The model under review builds one solid part; all positions refer to its coordinate system, in mm. A direction names the side the tool comes from. Coordinates: 2 decimals unless noted, no trailing zeros. Order: outer loops, then holes, each group sorted by start corner. A loop starts at its lowest first (then second) coordinate and runs counter-clockwise, first axis right, second up. Notation, with made-up numbers: (-11.5, 63.5) - (0.5, 63.5) arc R29 cw to (0.5, 100.5) - close; hole circle Ø2 at (-33.75, 2). An arc over 180 degrees is marked (long way). Answer in a Markdown table with one row per item.
Autodesk Inventor part; units mm, degrees
ref_plane "YZ Plane" through (0, 0, 0) normal (1, 0, 0) x (0, 1, 0)
ref_plane "XZ Plane" through (0, 0, 0) normal (0, 1, 0) x (-1, 0, 0)
ref_plane "XY Plane" through (0, 0, 0) normal (0, 0, 1) x (1, 0, 0)
sketch "Sketch1" plane through (0, 0, 0) normal (0, 0, 1) x (1, 0, 0)
  line L0 (2.5, 1.4434) -> (2.5, -1.4434)
  line L1 (2.5, -1.4434) -> (0, -2.8868)
  line L2 (0, -2.8868) -> (-2.5, -1.4434)
  line L3 (-2.5, -1.4434) -> (-2.5, 1.4434)
  line L4 (-2.5, 1.4434) -> (0, 2.8868)
  line L5 (0, 2.8868) -> (2.5, 1.4434)
  point P0 (0, 0)
  point P1 (0, 0)
  dimension "d0" = 5
extrude "Extrusion1" add sketch "Sketch1" along normal blind 26
sketch "Sketch2" plane through (0, 0, 26) normal (0, 0, 1) x (1, 0, 0)
  circle A0 centre (0, 0) radius 1.5
  dimension "d3" = 3
extrude "Extrusion2" add sketch "Sketch2" along normal blind 6
chamfer "Chamfer1" distance 0.5 angle 45 1 edges at (-1.5, 0, 32)
thread "Thread1"
sketch "Sketch3" plane through (0, 0, 0) normal (0, 0, -1) x (-1, 0, 0)
  point P0 (0, 0)
  point P1 (0, 0)
hole "Hole1" at (0, 0, 0) direction (0, 0, 1) diameter 2.459 depth 8.8 tip angle 118
properties part number "M3_26mm_Abstands"
Item 1: We need section A-A, the plane z = 10. Write out the cut boundary in (x, y).
Check values:
| item | result |
|---|---|
| outline | (-2.5, -1.44) - (0, -2.89) - (2.5, -1.44) - (2.5, 1.44) - (0, 2.89) - (-2.5, 1.44) - close |
Item 2: Mouldability with a two-part tool opening along X and no side actions: class faces 1 (the face through (-1.15, -1.24, 26)), 2 (the face through (0.064, 0.204, 9.41)), 3 (the face through (-1.233, -2.175, 12.818)) as +X half, -X half, draft (parallel to the pull), parting line (faces both ways), or undercut.
Check values:
| item | result |
|---|---|
| face 1 | draft |
| face 2 | undercut |
| face 3 | -X half |
Item 3: Tool access review of faces 4 (the face through (0.748, -0.976, 4.462)), 5 (the face through (1.267, -2.155, 12.818)), 6 (the face through (-1.5, -0.07, 28.71)): name each direction out of +Z, -Z, +X, -X, +Y, -Y from which nothing blocks a thin tool from reaching the whole face with its end or side.
Check values:
| item | result |
|---|---|
| face 4 | -Z |
| face 5 | +Z, -Z, +X, -Y |
| face 6 | +Z |
Item 4: Clearance check with a flat-ended pin moving along its axis: pin 1 Ø2 at (x, z) = (1.5, 25) entering from +Y. State where the tip first meets the part, or that it passes through.
Check values:
| item | result |
|---|---|
| pin 1 | y = 2.6 |
Item 5: To check wall thickness, follow line 1 (X direction, y = 0, z = 2.75); line 2 (Z direction, x = 1.85, y = -0.5); line 3 (Y direction, x = -0.75, z = 4). State the ranges of each line that lie inside material, in increasing order. Write a range as from..to.
Check values:
| item | result |
|---|---|
| line 1 | -2.5..-1.23, 1.23..2.5 |
| line 2 | 0..26 |
| line 3 | -2.45..-0.97, 0.97..2.45 |
Item 6: We need section B-B, the plane z = 28. Write out the cut boundary in (x, y), then the cut area to 3 significant figures.
Check values:
| item | result |
|---|---|
| outline | circle Ø3 at (0, 0) |
| area | 7.07 mm^2 |
